from build123d import *

# Parameters (mm, degrees)
SKETCH1_W           = 88.9
SKETCH1_H           = 184.762458854
SKETCH1_R           = 3.175
BOSS_EXTRUDE1_DEPTH = 3.175
FILLET1_R           = 5.08
FILLET2_R           = 12.7


with BuildPart() as part:
    # Sketch1 → Boss-Extrude1 (new body)
    with BuildSketch(Plane.XY):
        with Locations((1623.410721097, -4179.866189559)):
            Rectangle(SKETCH1_W, SKETCH1_H)
        with Locations((1598.010721097, -4106.534960132)):
            Circle(SKETCH1_R, mode=Mode.SUBTRACT)
        with BuildLine():
            Line((1648.810721097, -4168.715160172), (1611.515942217, -4114.879097445))
            ThreePointArc((1611.515942217, -4114.879097445), (1613.281788681, -4110.872023639), (1613.885721097, -4106.534960132))
            Line((1613.885721097, -4106.534960132), (1632.935721097, -4106.534960132))
            ThreePointArc((1632.935721097, -4106.534960132), (1637.585400946, -4117.760280283), (1648.810721097, -4122.409960132))
            Line((1648.810721097, -4122.409960132), (1648.810721097, -4168.715160172))
        make_face(mode=Mode.SUBTRACT)
        with BuildLine():
            ThreePointArc((1598.010721097, -4122.409960132), (1599.550748635, -4122.335084821), (1601.076248923, -4122.111165194))
            Line((1601.076248923, -4122.111165194), (1641.085877299, -4179.866189559))
            Line((1641.085877299, -4179.866189559), (1601.076248923, -4237.621213923))
            ThreePointArc((1601.076248923, -4237.621213923), (1599.550748635, -4237.397294297), (1598.010721097, -4237.322418986))
            Line((1598.010721097, -4237.322418986), (1598.010721097, -4122.409960132))
        make_face(mode=Mode.SUBTRACT)
        with BuildLine():
            ThreePointArc((1613.885721097, -4253.197418986), (1613.281788681, -4248.860355479), (1611.515942217, -4244.853281672))
            Line((1611.515942217, -4244.853281672), (1648.810721097, -4191.017218946))
            Line((1648.810721097, -4191.017218946), (1648.810721097, -4237.322418986))
            ThreePointArc((1648.810721097, -4237.322418986), (1637.585400946, -4241.972098834), (1632.935721097, -4253.197418986))
            Line((1632.935721097, -4253.197418986), (1613.885721097, -4253.197418986))
        make_face(mode=Mode.SUBTRACT)
        with Locations((1598.010721097, -4253.197418986)):
            Circle(SKETCH1_R, mode=Mode.SUBTRACT)
        with Locations((1648.810721097, -4106.534960132)):
            Circle(SKETCH1_R, mode=Mode.SUBTRACT)
        with Locations((1648.810721097, -4253.197418986)):
            Circle(SKETCH1_R, mode=Mode.SUBTRACT)
    extrude(amount=BOSS_EXTRUDE1_DEPTH)

    # Fillet1
    fillet1_edges = [part.edges().sort_by_distance(p)[0] for p in [
        (1648.810721097, -4191.017218946, 1.5875),
        (1641.085877299, -4179.866189559, 1.5875),
        (1648.810721097, -4168.715160172, 1.5875),
    ]]
    fillet(fillet1_edges, radius=FILLET1_R)

    # Fillet2
    fillet2_edges = [part.edges().sort_by_distance(p)[0] for p in [
        (1667.860721097, -4272.247418986, 1.5875),
        (1578.960721097, -4272.247418986, 1.5875),
        (1578.960721097, -4087.484960132, 1.5875),
        (1667.860721097, -4087.484960132, 1.5875),
    ]]
    fillet(fillet2_edges, radius=FILLET2_R)


solid = part.part
Can you work these out from the model? Positions are in its coordinate system, mm. A direction names the side the tool comes from. Give positions to 0.01 mm unless a question says otherwise; leave off trailing zeros. Order: outer loops, then holes, each group sorted by start corner. A loop starts at its lowest first (then second) coordinate and runs counter-clockwise, first axis right, second up. Notation, with made-up numbers: M 62,19 L 66,19 A16 cw 66,50 Z; hole C 0,77.5 d6. An arc over 180 degrees is marked long. Use a Markdown table: item, result. Add a question column.
Item 1: Suppose I cut it at D-D (y = -4213). List the corners of the cut face in (x, z) for me (3 decimals), then the cut area to 3 significant figures.
Item 2: Suppose I cut it at C-C (x = 1626.5). List the corners of the cut face in (y, z) for me (3 decimals).
Item 3: Suppose I cut it at B-B (y = -4161.5). List the corners of the cut face in (x, z) for me (3 decimals), then the cut area to 3 significant figures.
Item 4: For faces 4 (the cylindrical face through (1582.582, -4268.428, 1.61)), 5 (the cylindrical face through (1613.265, -4110.931, 1.565)), which set-ups out of +Z, -Z, +X, -X, +Y, -Y let a thin tool reach every point of the face, with its end or its side?
Item 5: If I drill on L1, parallel to Y at x = 1597.5, z = 2.3; L2, parallel to Y at x = 1645.5, z = 1.4; L3, parallel to Y at x = 1625, z = 1.7, over which ranges is the centre line in solid material (lowest first)? Write a range as [from, to].
Item 6: We'd pull the mould along Y, two halves only. Please class faces 1 (the cylindrical face through (1639.986, -4179.909, 1.61)), 2 (the flat face through (1667.861, -4181, 2)), 3 (the flat face through (1623, -4087.485, 2)): +Y half, -Y half, draft (parallel to the pull), parting line (faces both ways), or undercut.
Item 7: Suppose I cut it at A-A (z = 1.15). Count the separate pieces of the cut face and the enclosed holes in it, then the cut area to 3 significant figures.
Item 8: Will this pin go through, and if not, where does the flat tip stop? pin 1 (8.5 mm diameter, centred on x = 1598.01, y = -4253.2, fed in from +Z) (3 decimals).
Answer sheet:
| question | item | result |
|---|---|---|
| 1 | outline | M 1578.961,0 L 1598.011,0 L 1598.011,3.175 L 1578.961,3.175 Z; M 1618.133,0 L 1633.582,0 L 1633.582,3.175 L 1618.133,3.175 Z; M 1648.811,0 L 1667.861,0 L 1667.861,3.175 L 1648.811,3.175 Z |
| 1 | area | 170 mm² |
| 2 | outline | M -4272.247,0 L -4253.197,0 L -4253.197,3.175 L -4272.247,3.175 Z; M -4223.223,0 L -4200.921,0 L -4200.921,3.175 L -4223.223,3.175 Z; M -4158.811,0 L -4136.509,0 L -4136.509,3.175 L -4158.811,3.175 Z; M -4106.535,0 L -4087.485,0 L -4087.485,3.175 L -4106.535,3.175 Z |
| 3 | outline | M 1578.961,0 L 1598.011,0 L 1598.011,3.175 L 1578.961,3.175 Z; M 1628.363,0 L 1667.861,0 L 1667.861,3.175 L 1628.363,3.175 Z |
| 3 | area | 186 mm² |
| 4 | face 4 | +Z, -Z, -X, -Y |
| 4 | face 5 | +Z, -Z |
| 5 | L1 | y = [-4272.25, -4256.33], [-4250.06, -4109.67], [-4103.4, -4087.48] |
| 5 | L2 | y = [-4272.25, -4237.67], [-4202.51, -4157.22], [-4122.06, -4087.48] |
| 5 | L3 | y = [-4272.25, -4253.2], [-4225.39, -4203.09], [-4156.65, -4134.34], [-4106.53, -4087.48] |
| 6 | face 1 | undercut |
| 6 | face 2 | draft |
| 6 | face 3 | +Y half |
| 7 | separate pieces | 1 |
| 7 | enclosed holes | 7 |
| 7 | area | 11,400 mm² |
| 8 | pin 1 | stops at z = 3.175 |
